Could you check a few things on this model? Use its own coordinates, in mm. A direction names the side the tool comes from. Give positions to 0.01 mm unless a question says otherwise; leave off trailing zeros. Loops run counter-clockwise (first coordinate to the right, second up) from the corner with the lowest first, then second, coordinate; pieces in that order, holes last. Notation, with made-up numbers: M 44,-9.5 L 61,-9.5 A14 cw 61,-2.5 Z; hole C 22.5,-33.75 d3. An arc over 180 degrees is marked long. Return JSON: item names as keys, results as strings. Group by question number.
1. If we section it at C-C (y = -27.5): Write out the boundary of the cut face in (x, z).
2. Please list where these lines run through material, in increasing order: line 1 (X direction, y = -43, z = -0.7); line 2 (X direction, y = -52, z = -0.8); line 3 (Y direction, x = 17, z = -0.65).
3. If we mould it in two halves opening along X, with no side actions, what happens to faces 3 (the flat face through (-22, -41, 0)), 4 (the flat face through (50.5, -37, 0))? For each: +X half, -X half, draft (parallel to the pull), parting line (faces both ways), or undercut.
4. If we section it at A-A (y = -36.5): Write out the boundary of the cut face in (x, z).
5. For faces 1 (the flat face through (-22, -29, 0)), 2 (the flat face through (-20, -10, 0)), which set-ups out of +Z, -Z, +X, -X, +Y, -Y let a thin tool reach every point of the face, with its end or its side?
6. If we section it at B-B (x = 18): Write out the boundary of the cut face in (y, z), plus the area to 3 significant figures.
7. If we section it at D-D (z = -0.55): State how many separate pieces and enclosed holes the cut face has, plus the area to 3 significant figures.
8. For pin 1 (0.9 mm diameter, centred on x = 17, z = -0.5, fed in from +Y); pin 2 (1.5 mm diameter, centred on x = 30.5, z = -0.5, fed in from +Y), each with a flat end and sliding along its axis, tell me the tip position at first contact or that it passes through.
```python
from build123d import *

# Parameters (mm, degrees)
SKETCH1_W           = 101
SKETCH1_H           = 58.2
BOSS_EXTRUDE1_DEPTH = 1.5
SKETCH2_W           = 6
SKETCH2_H           = 6
SKETCH2_W_2         = 40
SKETCH2_H_2         = 8
SKETCH2_W_3         = 34
SKETCH2_H_3         = 10
CUT_EXTRUDE2_DEPTH  = 83.840871555


with BuildPart() as part:
    # Sketch1 → Boss-Extrude1 (new, symmetric)
    with BuildSketch(Plane.XY):
        with Locations((0, -36.5)):
            Rectangle(SKETCH1_W, SKETCH1_H)
    extrude(amount=BOSS_EXTRUDE1_DEPTH, both=True)

    # Sketch2 → Cut-Extrude2 (cut, through all)
    with BuildSketch(Plane.XY.offset(1.5)):
        with Locations((16, -34.713248654)):
            Rectangle(SKETCH2_W, SKETCH2_H)
        with Locations((31.881445826, -41.57558602)):
            Rectangle(SKETCH2_W, SKETCH2_H)
        with Locations((0, -10.4)):
            Rectangle(SKETCH2_W_2, SKETCH2_H)
        with Locations((16, -53.6)):
            Rectangle(SKETCH2_W, SKETCH2_H)
        Polygon((-22, -43.6), (-16, -43.6), (-16, -37.6), (-10, -37.6), (-10, -31.6), (-16, -31.6), (-16, -25.6), (-22, -25.6), (-22, -31.6), (-28, -31.6), (-28, -37.6), (-22, -37.6), align=None)
        with Locations((30, -10.07558602)):
            Rectangle(SKETCH2_W, SKETCH2_H_2)
        with Locations((-19, -55.6)):
            Rectangle(SKETCH2_W_3, SKETCH2_H_3)
    extrude(amount=-CUT_EXTRUDE2_DEPTH, mode=Mode.SUBTRACT)


solid = part.part
```
Answer:
{
 "1": {"outline": "M -50.5,-1.5 L -22,-1.5 L -22,1.5 L -50.5,1.5 Z; M -16,-1.5 L 50.5,-1.5 L 50.5,1.5 L -16,1.5 Z"},
 "2": {"line 1": "x = -50.5 to -22, -16 to 28.88, 34.88 to 50.5", "line 2": "x = -50.5 to -36, -2 to 13, 19 to 50.5", "line 3": "y = -65.6 to -56.6, -50.6 to -37.71, -31.71 to -13.4"},
 "3": {"face 3": "undercut", "face 4": "+X half"},
 "4": {"outline": "M -50.5,-1.5 L -28,-1.5 L -28,1.5 L -50.5,1.5 Z; M -10,-1.5 L 13,-1.5 L 13,1.5 L -10,1.5 Z; M 19,-1.5 L 50.5,-1.5 L 50.5,1.5 L 19,1.5 Z"},
 "5": {"face 1": "+Z, -Z", "face 2": "+Z, -Z, +Y"},
 "6": {"outline": "M -65.6,-1.5 L -56.6,-1.5 L -56.6,1.5 L -65.6,1.5 Z; M -50.6,-1.5 L -37.71,-1.5 L -37.71,1.5 L -50.6,1.5 Z; M -31.71,-1.5 L -13.4,-1.5 L -13.4,1.5 L -31.71,1.5 Z", "area": "121 mm²"},
 "7": {"separate pieces": "1", "enclosed holes": "5", "area": "4,970 mm²"},
 "8": {"pin 1": "stops at y = -13.4", "pin 2": "stops at y = -14.08"}
}
